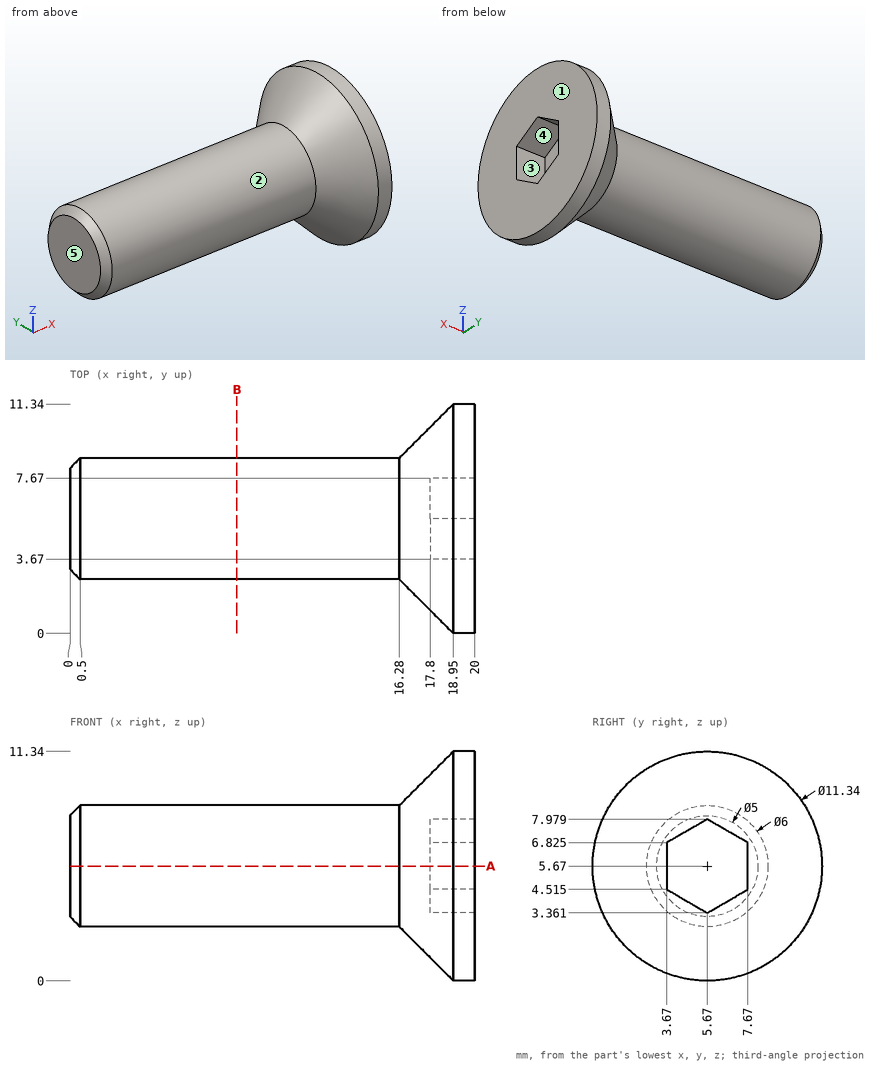
Study the drawing (mm; zero at the part's minimum x, y, z) and answer. A direction names the side the tool comes from. Coordinates: 2 decimals unless noted, no trailing zeros. Write each loop counter-clockwise with the first axis right and the second up, starting at its lowest first coordinate (ties: lowest second). Pieces come first, ordered by that corner, then holes. Notation, with made-up numbers: (23, 6) - (63, 6) arc R37 cw to (63, 45) - close; hole circle Ø11 at (76.25, -36.75). An arc over 180 degrees is marked (long way). Answer as a JSON object with one key per item and string values.
Q1. Which of the six approach directions +Z, -Z, +X, -X, +Y, -Y give full straight-line access (tool end or side, diameter ignored) to the marked faces 4 and 5?
Results list:
{"face 4": "+X", "face 5": "+Z, -Z, -X, +Y, -Y"}
Q2. For a pull along Z with two mould halves and no side action, classify the marked faces 1, 2 and 3 as pulls with the +Z half, pulls with the -Z half, needs draft (parallel to the pull), parting line crosses it, or undercut.
Results list:
{"face 1": "needs draft", "face 2": "parting line crosses it", "face 3": "undercut"}
Q3. Find section A-A (z = 5.67). Write down the section's boundary in (x, y), plus the area to 3 significant figures.
Results list:
{"outline": "(0, 3.17) - (0.5, 2.67) - (16.28, 2.67) - (18.95, 0) - (20, 0) - (20, 3.67) - (17.8, 3.67) - (17.8, 7.67) - (20, 7.67) - (20, 11.34) - (18.95, 11.34) - (16.28, 8.67) - (0.5, 8.67) - (0, 8.17) - close", "area": "124 mm^2"}
Q4. Given pin 1 Ø1.2 at (y, z) = (6, 5) entering from +X; pin 2 Ø2 at (x, z) = (6, 7.5) entering from +Y; pin 3 Ø3 at (x, y) = (6, 6.5) entering from -Z, each flat-ended and moving along its own axis, determine where each tip first touches the part or whether it passes through.
Results list:
{"pin 1": "stops at x = 17.8", "pin 2": "stops at y = 8.55", "pin 3": "stops at z = 2.67"}
Q5. Find section B-B (x = 8.25). Write down the section's boundary in (y, z), plus the area to 3 significant figures.
Results list:
{"outline": "circle Ø6 at (5.67, 5.67)", "area": "28.3 mm^2"}
Q6. Consider L1, parallel to Z at x = 15, y = 5.5 (1 decimal); L2, parallel to Y at x = 18.75, z = 9.5 (1 decimal); L3, parallel to Y at x = 5.75, z = 3 (1 decimal). Determine where each line is inside the solid, lowest interval first. Write a range as from..to.
Results list:
{"L1": "z = 2.7..8.7", "L2": "y = 1.8..9.6", "L3": "y = 4.3..7"}
